Source: three-view drawing plus pictorial views. Frame: mm from the lowest corner of the part. Give positions to 0.01 mm unless a question says otherwise; leave off trailing zeros. Loops run counter-clockwise (first coordinate to the right, second up) from the corner with the lowest first, then second, coordinate; pieces in that order, holes last.
1. Section A-A, the plane x = 69. Output: boundary loops of the cut face in (y, z), then the cut area to 3 significant figures.
2. First-contact query: P1, Ø4, axis at x = 35.5, z = 55.5, coming from the -Y side; P2, Ø5, axis at x = 174, y = 7, coming from the -Z side; P3, Ø6, axis at x = 173.5, y = 3, coming from the +Z side. Flat tips, straight axial feed; report the tip coordinate or a pass-through.
3. Section C-C, the plane y = 5.5. Output: boundary loops of the cut face in (x, z), then the cut area to 3 significant figures.
4. Material intervals for line 1 along Z through (x, y) = (172, 7.75); line 2 along Z through (x, y) = (99.5, 2.5); line 3 along X through (y, z) = (4.75, 204), sorted ascending.
5. Section B-B, the plane z = 179. Output: boundary loops of the cut face in (x, y), then the cut area to 3 significant figures.
6. Section D-D, the plane x = 201.5. Output: boundary loops of the cut face in (y, z), then the cut area to 3 significant figures.
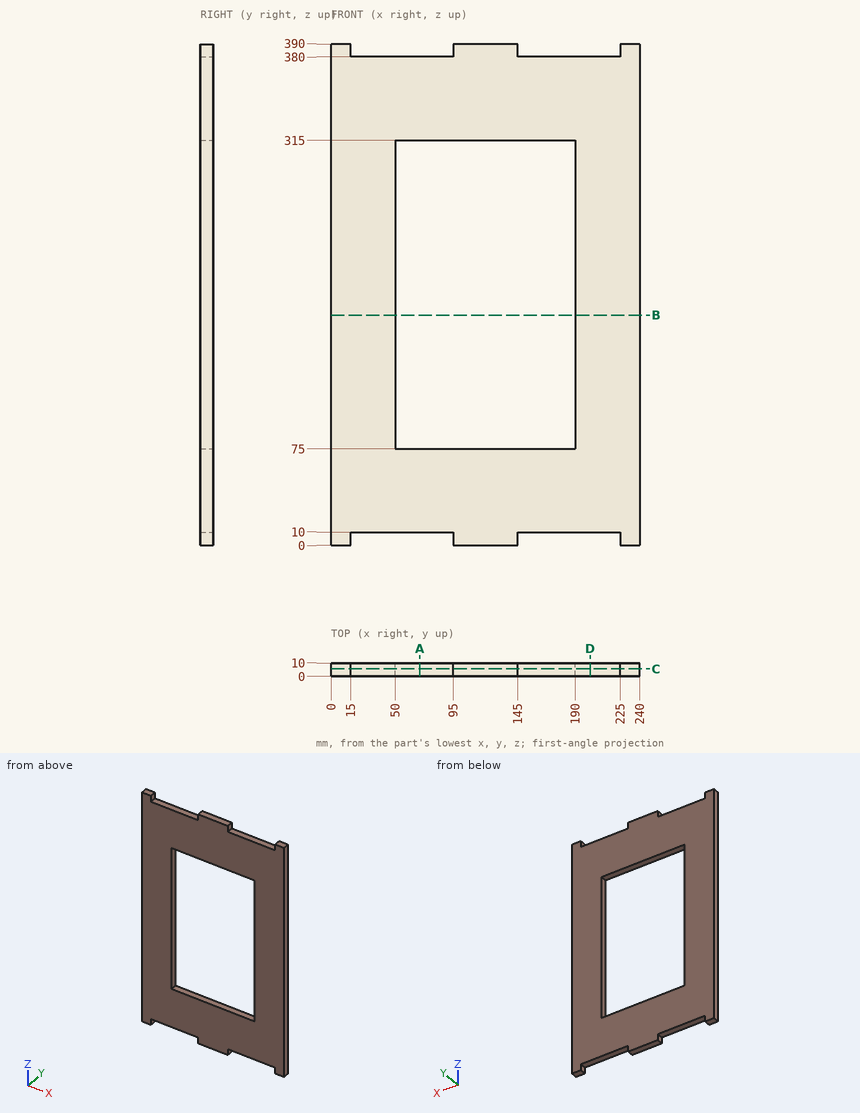
Answers below:
1. outline: (0, 10) - (10, 10) - (10, 75) - (0, 75) - close; (0, 315) - (10, 315) - (10, 380) - (0, 380) - close
1. area: 1,300 mm2
2. P1: stops at y = 0
2. P2: stops at z = 10
2. P3: stops at z = 380
3. outline: (0, 0) - (15, 0) - (15, 10) - (95, 10) - (95, 0) - (145, 0) - (145, 10) - (225, 10) - (225, 0) - (240, 0) - (240, 390) - (225, 390) - (225, 380) - (145, 380) - (145, 390) - (95, 390) - (95, 380) - (15, 380) - (15, 390) - (0, 390) - close; hole (50, 75) - (190, 75) - (190, 315) - (50, 315) - close
3. area: 56,800 mm2
4. line 1: z = 10 to 75, 315 to 380
4. line 2: z = 0 to 75, 315 to 390
4. line 3: x = 0 to 50, 190 to 240
5. outline: (0, 0) - (50, 0) - (50, 10) - (0, 10) - close; (190, 0) - (240, 0) - (240, 10) - (190, 10) - close
5. area: 1,000 mm2
6. outline: (0, 10) - (10, 10) - (10, 380) - (0, 380) - close
6. area: 3,700 mm2
